Verification items for the finished model (mm, model axes). A direction names the side the tool comes from. Give positions to 0.01 mm unless a question says otherwise; leave off trailing zeros. Write each loop counter-clockwise with the first axis right and the second up, starting at its lowest first coordinate (ties: lowest second). Pieces come first, ordered by that corner, then holes. Notation, with made-up numbers: (-6.75, 28.25) - (2.25, 28.25) arc R20 cw to (2.25, 45.25) - close; hole circle Ø5 at (-16.5, 89). An arc over 180 degrees is marked (long way). Put each result on its own line as item: value.
Autodesk Inventor part; units mm, degrees
ref_plane "YZ Plane" through (0, 0, 0) normal (1, 0, 0) x (0, 1, 0)
ref_plane "XZ Plane" through (0, 0, 0) normal (0, 1, 0) x (-1, 0, 0)
ref_plane "XY Plane" through (0, 0, 0) normal (0, 0, 1) x (1, 0, 0)
sketch "Skizze1" plane through (0, 0, 0) normal (0, 0, 1) x (1, 0, 0)
  line L0 (-76.5, 0) -> (76.5, 0)
  line L1 (76.5, 0) -> (76.5, 306.5)
  line L2 (76.5, 306.5) -> (-76.5, 306.5)
  line L3 (-76.5, 306.5) -> (-76.5, 0)
  line L4 (75, 306.5) -> (75, 0) construction
  line L5 (-75, 0) -> (-75, 306.5) construction
  line L6 (-76.5, 305) -> (76.5, 305) construction
  point P0 (0, 0)
  point P1 (0, 0)
  point P2 (-75, 305)
  point P3 (75, 305)
  dimension "d2" = 1.5
  dimension "d3" = 1.5
  dimension "d4" = 1.5
  dimension "d5" = 150
  dimension "d6" = 305
extrude "Bodenplatte" add sketch "Skizze1" along normal blind 1.8
sketch "Skizze3" plane through (0, 0, 1.8) normal (0, 0, 1) x (1, 0, 0)
  line L0 (-76.5, 306.5) -> (-76.5, 0)
  line L1 (-76.5, 0) -> (76.5, 0)
  line L2 (-76.5, 306.5) -> (-75, 306.5)
  line L3 (-75, 306.5) -> (-75, 0)
  line L4 (-75, 0) -> (-76.5, 0)
  line L5 (-76.5, 0) -> (-76.5, 306.5)
  point P0 (0, 0)
  dimension "d9" = 1.5
extrude "Wand_links" add sketch "Skizze3" along normal blind 180
sketch "Skizze4" plane through (0, 0, 1.8) normal (0, 0, 1) x (1, 0, 0)
  line L0 (76.5, 0) -> (76.5, 306.5)
  line L1 (76.5, 0) -> (75, 0)
  line L2 (75, 0) -> (75, 306.5)
  line L3 (75, 306.5) -> (76.5, 306.5)
  line L4 (76.5, 306.5) -> (76.5, 0)
  point P0 (0, 0)
  dimension "d12" = 1.5
extrude "Wand_rechts" add sketch "Skizze4" along normal blind 180
sketch "Skizze5" plane through (0, 0, 1.8) normal (0, 0, 1) x (1, 0, 0)
  line L0 (75, 306.5) -> (-75, 306.5)
  line L1 (75, 306.5) -> (75, 0)
  line L2 (-75, 0) -> (-75, 306.5)
  line L3 (-75, 306.5) -> (-76.5, 306.5)
  line L4 (-75, 306.5) -> (75, 306.5)
  line L5 (75, 306.5) -> (75, 305)
  line L6 (75, 305) -> (-75, 305)
  line L7 (-75, 305) -> (-75, 306.5)
  point P0 (0, 0)
  dimension "d15" = 1.5
extrude "Wand_vorn" add sketch "Skizze5" along normal blind 180
sketch "Skizze6" plane through (-76.5, 306.5, 0) normal (0, 1, 0) x (1, 0, 0)
  line L0 (153, 0) -> (0, 0) construction
  line L1 (0, 0) -> (0, -181.8) construction
  line L2 (153, -181.8) -> (0, -181.8) construction
  line L3 (153, 0) -> (153, -181.8) construction
  line L4 (115.5, -147.2) -> (37.5, -147.2)
  line L5 (36.3, -146) -> (36.3, -103)
  line L6 (37.5, -101.8) -> (115.5, -101.8)
  line L7 (116.7, -103) -> (116.7, -146)
  line L8 (76.5, 0) -> (76.5, -181.8) construction
  line L9 (153, 0) -> (153, -181.8) construction
  line L10 (151.5, -1.8) -> (1.5, -1.8) construction
  arc A0 (115.5, -147.2) -> (116.7, -146) centre (115.5, -146) ccw
  arc A1 (36.3, -146) -> (37.5, -147.2) centre (37.5, -146) ccw
  arc A2 (37.5, -101.8) -> (36.3, -103) centre (37.5, -103) ccw
  arc A3 (116.7, -103) -> (115.5, -101.8) centre (115.5, -103) ccw
  point P0 (116.7, -147.2)
  point P1 (36.3, -101.8)
  point P2 (36.3, -147.2)
  point P3 (116.7, -101.8)
  point P4 (76.5, -147.2)
  dimension "d18" = 80.4
  dimension "d19" = 45.4
  dimension "d25" = 100
  dimension "d35" = 1.2
extrude "Fenster_vorn" cut sketch "Skizze6" against normal up to next
sketch "Skizze7" plane through (76.5, 0, 0) normal (1, 0, 0) x (0, 0, -1)
  line L0 (-1.8, 0) -> (-1.8, 305) construction
  line L1 (-181.8, 305) -> (-1.8, 305) construction
  line L2 (-146, 112.3) -> (-103, 112.3)
  line L3 (-101.8, 113.5) -> (-101.8, 191.5)
  line L4 (-103, 192.7) -> (-146, 192.7)
  line L5 (-147.2, 191.5) -> (-147.2, 113.5)
  arc A0 (-147.2, 113.5) -> (-146, 112.3) centre (-146, 113.5) ccw
  arc A1 (-146, 192.7) -> (-147.2, 191.5) centre (-146, 191.5) ccw
  arc A2 (-101.8, 191.5) -> (-103, 192.7) centre (-103, 191.5) ccw
  arc A3 (-103, 112.3) -> (-101.8, 113.5) centre (-103, 113.5) ccw
  line L6 (-1.8, 152.5) -> (-181.8, 152.5) construction
  line L7 (-181.8, 0) -> (-181.8, 305) construction
  point P0 (0, 0)
  point P1 (-101.8, 192.7)
  point P2 (-101.8, 112.3)
  point P3 (-147.2, 192.7)
  point P4 (-147.2, 152.5)
  dimension "d26" = 45.4
  dimension "d27" = 80.4
  dimension "d28" = 1.2
  dimension "d29" = 1.2
  dimension "d30" = 1.2
  dimension "d31" = 1.2
  dimension "d34" = 100
extrude "Fenster_rechts" cut sketch "Skizze7" against normal blind 10
sketch "Skizze8" plane through (76.5, 0, 0) normal (1, 0, 0) x (0, 0, -1)
  line L0 (-181.8, 305) -> (-1.8, 305) construction
  line L1 (-1.8, 0) -> (-1.8, 305) construction
  line L2 (-166.8, 235) -> (-1.8, 235)
  line L3 (-1.8, 235) -> (-1.8, 300)
  line L4 (-1.8, 300) -> (-166.8, 300)
  line L5 (-166.8, 300) -> (-166.8, 235)
  point P0 (0, 0)
  dimension "d36" = 65
  dimension "d37" = 165
  dimension "d38" = 5
extrude "Tuer_rechts" cut sketch "Skizze8" against normal blind 10
properties part number "Koffer_leer"
Q1. Scan lines: line 1 along X through (y, z) = (186, 82); line 2 along Y through (x, z) = (-66.5, 19.5); line 3 along X through (y, z) = (136.5, 127). Record each from-to range of solid material in increasing order.
Answers follow:
line 1: x = -76.5 to -75, 75 to 76.5
line 2: y = 305 to 306.5
line 3: x = -76.5 to -75
Q2. Release check for a two-part mould opening along X. For faces 3 (the face through (75, 116, 91)), 4 (the face through (-1, 155, 0)), 5 (the face through (-76.5, 155, 90)), 6 (the face through (1, 305, 91)) record: released by +X, released by -X, zero draft, split by the parting line, or undercut.
Answers follow:
face 3: undercut
face 4: zero draft
face 5: released by -X
face 6: undercut
Q3. Go/stop test with a flat-tipped pin: pin 1 Ø10 at (x, y) = (35.5, 139.5) entering from +Z. Record where the tip stops, or that it passes through.
Answers follow:
pin 1: stops at z = 1.8
Q4. Section check A-A, the plane z = 35.5. Record the cut outline in (x, y), plus the area to 3 significant figures.
Answers follow:
outline: (-76.5, 0) - (-75, 0) - (-75, 305) - (75, 305) - (75, 300) - (76.5, 300) - (76.5, 306.5) - (-76.5, 306.5) - close; (75, 0) - (76.5, 0) - (76.5, 235) - (75, 235) - close
area: 1,050 mm2
Q5. Section check C-C, the plane x = -22.5. Record the cut outline in (y, z).
Answers follow:
outline: (0, 0) - (306.5, 0) - (306.5, 101.8) - (305, 101.8) - (305, 1.8) - (0, 1.8) - close; (305, 147.2) - (306.5, 147.2) - (306.5, 181.8) - (305, 181.8) - close
Q6. Section check B-B, the plane y = 179. Record the cut outline in (x, z), plus the area to 3 significant figures.
Answers follow:
outline: (-76.5, 0) - (76.5, 0) - (76.5, 101.8) - (75, 101.8) - (75, 1.8) - (-75, 1.8) - (-75, 181.8) - (-76.5, 181.8) - close; (75, 147.2) - (76.5, 147.2) - (76.5, 181.8) - (75, 181.8) - close
area: 747 mm2
Q7. Section check D-D, the plane y = 67.5. Record the cut outline in (x, z).
Answers follow:
outline: (-76.5, 0) - (76.5, 0) - (76.5, 181.8) - (75, 181.8) - (75, 1.8) - (-75, 1.8) - (-75, 181.8) - (-76.5, 181.8) - close
Q8. Set-up check for faces 1 (the face through (1, 306.5, 90)), 2 (the face through (-75, 155, 91)): record each of +Z, -Z, +X, -X, +Y, -Y from which the full face is reachable in a straight line by a thin tool's end or side.
Answers follow:
face 1: +Z, -Z, +X, -X, +Y
face 2: +Z, -Y
